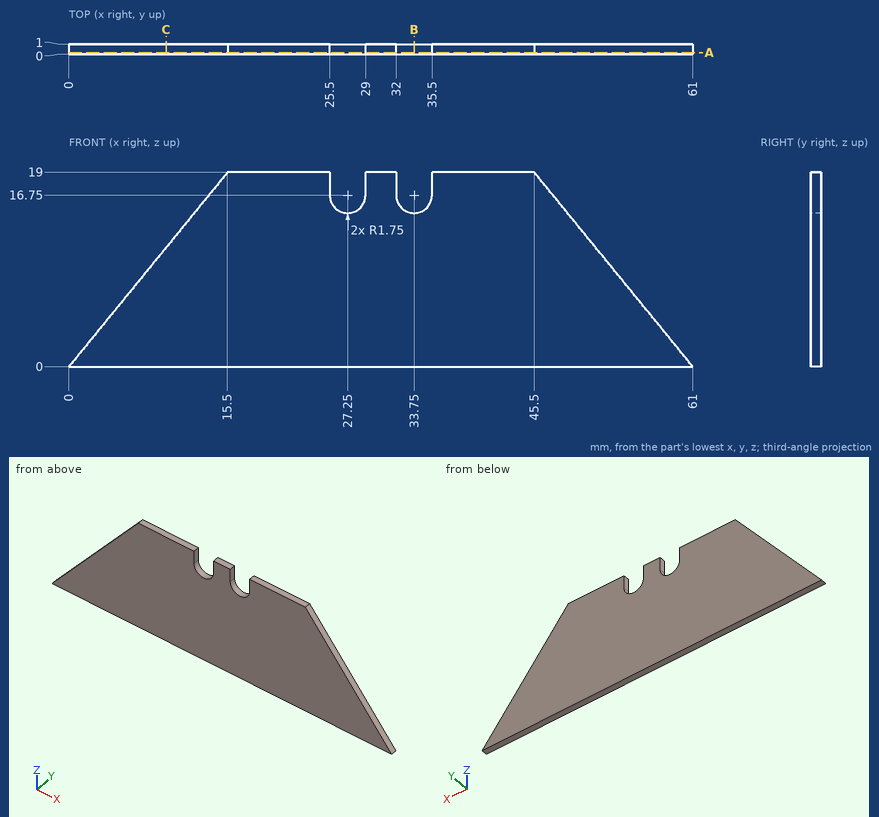
Design review of the part shown in the three views and the two pictorial views. Dimensions are in mm from the part's minimum x, y and z. Coordinates: 2 decimals unless noted, no trailing zeros. Write each loop counter-clockwise with the first axis right and the second up, starting at its lowest first coordinate (ties: lowest second). Pieces come first, ordered by that corner, then holes.
1) We need section B-B on x = 33.75. State the section outline as (y, z) points.
2) To check wall thickness, follow probe 1 along X at (y, z) = (0.3, 16); probe 2 along Z at (x, y) = (10, 0.4); probe 3 along Z at (x, y) = (49.5, 0.15). State the ranges of each line that lie inside material, in increasing order.
3) We need section C-C on x = 9.5. State the section outline as (y, z) points, then the cut area to 3 significant figures.
4) We need section A-A on y = 0.15. State the section outline as (x, z) points.
Answer list:
1. outline: (0, 0) - (1, 0) - (1, 15) - (0, 15) - close
2. probe 1: x = 13.05 to 25.67, 28.83 to 32.17, 35.33 to 47.95
2. probe 2: z = 0 to 12.26
2. probe 3: z = 0 to 14.1
3. outline: (0, 0) - (1, 0) - (1, 11.65) - (0, 11.65) - close
3. area: 11.6 mm2
4. outline: (0, 0) - (61, 0) - (45.5, 19) - (35.5, 19) - (35.5, 16.75) arc R1.75 cw to (32, 16.75) - (32, 19) - (29, 19) - (29, 16.75) arc R1.75 cw to (25.5, 16.75) - (25.5, 19) - (15.5, 19) - close
